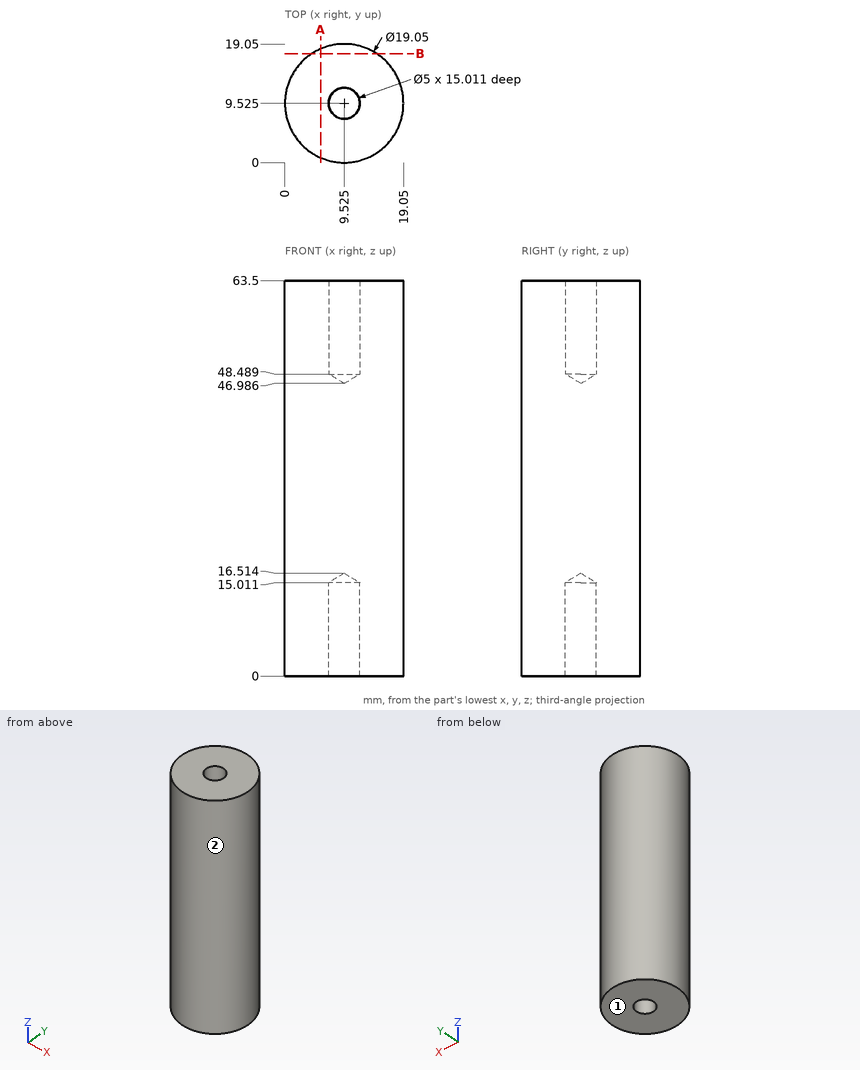
Job drawing, mm, ordinate dimensions from the low corner. One solid piece. Give positions to 0.01 mm unless a question says otherwise; leave off trailing zeros. Write each loop counter-clockwise with the first axis right and the second up, starting at its lowest first coordinate (ties: lowest second). Pieces come first, ordered by that corner, then holes. Notation, with made-up numbers: M 88,35.5 L 120,35.5 A11 cw 120,41.5 Z; hole C 23.25,36 d2. An arc over 180 degrees is marked long. One line per item, written item: value. Start each with the question number.
Q1. Saw through at B-B, the plane y = 17.5. Write the cut outline in (x, z).
Q2. Drop flat-ended pins along their axis: pin 1 Ø2 at (x, z) = (16.5, 45.5) entering from +Y; pin 2 Ø4 at (x, y) = (9.5, 4) entering from -Z; pin 3 Ø2 at (x, z) = (5.5, 16.5) entering from -Y; pin 4 Ø3 at (x, y) = (9.525, 9.525) entering from -Z. Give the stop position or say it passes through.
Q3. Two-plate mould, pull along X, no slides. Class the marked faces 1 and 2: +X half, -X half, draft (parallel to the pull), parting line (faces both ways), or undercut.
Q4. Probe probe 1 along X at (y, z) = (10, 53.5); probe 2 along X at (y, z) = (13.5, 6.5); probe 3 along Z at (x, y) = (10, 11.75) (1 decimal). List the from-to ranges inside material, lowest first. Write a range as [from, to].
Q5. Saw through at A-A, the plane x = 5.75. Write the cut outline in (y, z).
Output values:
1. outline: M 4.32,0 L 14.73,0 L 14.73,63.5 L 4.32,63.5 Z
2. pin 1: stops at y = 16.94
2. pin 2: stops at z = 0
2. pin 3: stops at y = 0.49
2. pin 4: stops at z = 15.61
3. face 1: draft
3. face 2: parting line
4. probe 1: x = [0.01, 7.07], [11.98, 19.04]
4. probe 2: x = [0.87, 18.18]
4. probe 3: z = [15.1, 48.4]
5. outline: M 0.78,0 L 18.27,0 L 18.27,63.5 L 0.78,63.5 Z
